Could you check a few things on this drawing? It's one solid part, dimensions in mm from its lowest x, y, z. Give positions to 0.01 mm unless a question says otherwise; leave off trailing zeros. Loops run counter-clockwise (first coordinate to the right, second up) from the corner with the lowest first, then second, coordinate; pieces in that order, holes last. Notation, with made-up numbers: (-11, 62) - (-5, 62) arc R21 ccw to (-5, 69) - close; hole circle Ø3 at (3.25, 62.25). An arc over 180 degrees is marked (long way). Answer as a JSON object with one key per item and string values.
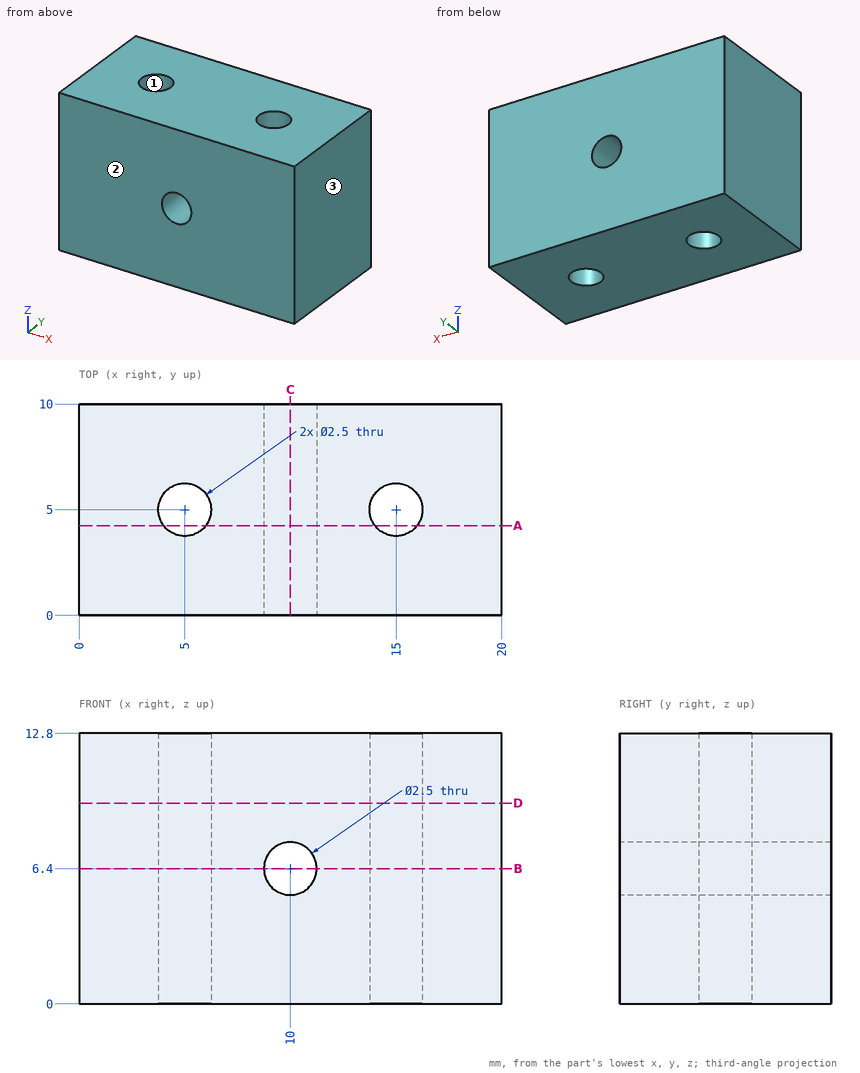
1) I'm going to push a flat-ended pin straight in: P1, Ø2, axis at x = 15, y = 5, coming from the +Z side. Where does the tip first touch, or does it pass through?
Check sheet entries:
{"P1": "through"}
2) Imagine slicing it at C-C on x = 10. Write out the boundary of the cut face in (y, z).
Check sheet entries:
{"outline": "(0, 0) - (10, 0) - (10, 5.15) - (0, 5.15) - close; (0, 7.65) - (10, 7.65) - (10, 12.8) - (0, 12.8) - close"}
3) Imagine slicing it at D-D on z = 9.5. Write out the boundary of the cut face in (x, y), and give its area (3 significant figures).
Check sheet entries:
{"outline": "(0, 0) - (20, 0) - (20, 10) - (0, 10) - close; hole circle Ø2.5 at (5, 5); hole circle Ø2.5 at (15, 5)", "area": "190 mm2"}
4) Imagine slicing it at A-A on y = 4.25. Write out the boundary of the cut face in (x, z), and give its area (3 significant figures).
Check sheet entries:
{"outline": "(0, 0) - (4, 0) - (4, 12.8) - (0, 12.8) - close; (6, 0) - (14, 0) - (14, 12.8) - (6, 12.8) - close; (16, 0) - (20, 0) - (20, 12.8) - (16, 12.8) - close; hole circle Ø2.5 at (10, 6.4)", "area": "200 mm2"}
5) If we mould it in two halves opening along Y, with no side actions, what happens to the marked faces 1, 2 and 3? For each: released by +Y, released by -Y, zero draft, split by the parting line, or undercut.
Check sheet entries:
{"face 1": "undercut", "face 2": "released by -Y", "face 3": "zero draft"}
6) Imagine slicing it at B-B on z = 6.4. Write out the boundary of the cut face in (x, y), and give its area (3 significant figures).
Check sheet entries:
{"outline": "(0, 0) - (8.75, 0) - (8.75, 10) - (0, 10) - close; (11.25, 0) - (20, 0) - (20, 10) - (11.25, 10) - close; hole circle Ø2.5 at (5, 5); hole circle Ø2.5 at (15, 5)", "area": "165 mm2"}
7) I need wall thicknesses on L1, parallel to X at y = 5, z = 9.75; L2, parallel to Y at x = 15, z = 5.5; L3, parallel to Z at x = 10, y = 7.75. Which ranges of each line are inside material? Lowest first, please.
Check sheet entries:
{"L1": "0 to 3.75, 6.25 to 13.75, 16.25 to 20", "L2": "0 to 3.75, 6.25 to 10", "L3": "0 to 5.15, 7.65 to 12.8"}
